Model file for the job. Use its own axes, mm. Face numbers are marked on the shaded views. Round coordinates to 2 decimals unless told otherwise and drop trailing zeros. Loops run counter-clockwise (first coordinate to the right, second up) from the corner with the lowest first, then second, coordinate; pieces in that order, holes last. Notation, with made-up numbers: M -26.75,36.5 L 6.25,36.5 A8 cw 6.25,41.5 Z; hole C -15.75,50 d10. An arc over 180 degrees is marked long. Use a Markdown table: item, result. Add a question column.
Q1. Mould opens along Z. For the marked faces 1 and 2 say: +Z half, -Z half, draft (parallel to the pull), parting line (faces both ways), or undercut.
Q2. Cut at B-B (z = 0). Give the cut face in (x, y), plus the area to 3 significant figures.
Q3. Probe line 1 (Z direction, x = -9, y = 4.25); line 2 (X direction, y = 4.7, z = 0); line 3 (Y direction, x = -38, z = -9). List the from-to ranges inside material, lowest first. Write a range as from..to.
Q4. Pin check, flat tips, straight feed: pin 1 (2.5 mm diameter, centred on y = 12, z = -6.5, fed in from +X); pin 2 (3.5 mm diameter, centred on x = -18.5, y = 4, fed in from -Z); pin 3 (5 mm diameter, centred on y = 3.5, z = 20, fed in from +X); pin 4 (1.5 mm diameter, centred on x = -40.5, z = -1, fed in from -Y). Stop position of each tip, or through.
Q5. Cut at A-A (x = 61.3). Give the cut face in (y, z), plus the area to 3 significant figures.
Q6. Cut at C-C (z = 61.3). Give the cut face in (x, y).
Q7. Cut at D-D (x = 0). Give the cut face in (y, z).
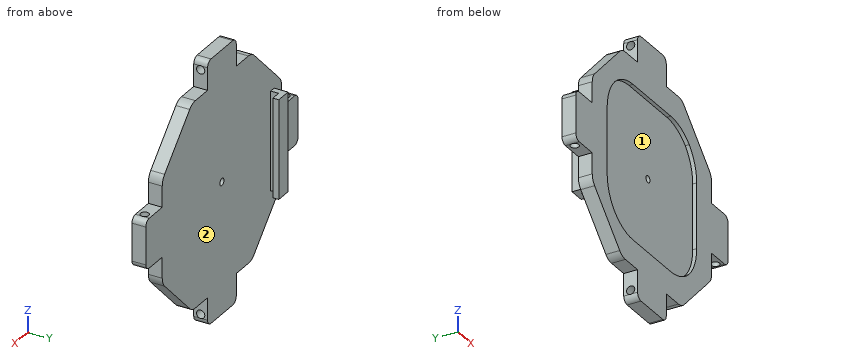
from build123d import *

# Parameters (mm, degrees)
SKETCH_1_W          = 14.3
SKETCH_1_H          = 25
SKETCH_1_W_2        = 25
SKETCH_1_H_2        = 14.3
EXTRUDE_1_DEPTH     = 7
FILLET_1_R          = 3
FILLET_2_R          = 7
FILLET_3_R          = 23
EXTRUDE_START       = -5
EXTRUDE_2_DEPTH     = 5
SKETCH_7_R          = 1.75
CUT_EXTRUDE_5_DEPTH = 95.023294986
SKETCH_9_W          = 3
SKETCH_9_H          = 50
EXTRUDE_3_DEPTH     = 7
SKETCH_10_W         = 50
SKETCH_10_H         = 3
EXTRUDE_4_DEPTH     = 5
SKETCH_11_R         = 2.1
CUT_EXTRUDE_6_DEPTH = 104.928485027
SKETCH_12_R         = 2.1
CUT_EXTRUDE_7_DEPTH = 104.928485103


with BuildPart() as part:
    # 스케치1 → 보스-돌출1 (new body)
    with BuildSketch(Plane(origin=(0, 0, 0), x_dir=(1, 0, 0), z_dir=(0, 1, 0))):
        Polygon((-26, 52), (-39, 39), (-26, 39), (26, 39), (39, 39), (26, 52), (12.5, 52), (-12.5, 52), align=None)
        Polygon((-26, 39), (-39, 39), (-39, 26), align=None)
        Polygon((-39, 26), (-39, 39), (-52, 26), (-52, 12.5), (-52, -12.5), (-52, -26), (-39, -39), (-39, -26), align=None)
        with Locations((-59.15, 0)):
            Rectangle(SKETCH_1_W, SKETCH_1_H)
        with Locations((0, 59.15)):
            Rectangle(SKETCH_1_W_2, SKETCH_1_H_2)
        Polygon((39, 39), (26, 39), (39, 26), align=None)
        Polygon((52, 26), (39, 39), (39, 26), (39, -26), (39, -39), (52, -26), (52, -12.5), (52, 12.5), align=None)
        with Locations((59.15, 0)):
            Rectangle(SKETCH_1_W, SKETCH_1_H)
        Polygon((39, -39), (39, -26), (26, -39), align=None)
        Polygon((-26, -39), (-39, -39), (-26, -52), (-12.5, -52), (12.5, -52), (26, -52), (39, -39), (26, -39), align=None)
        Polygon((-26, -39), (-39, -26), (-39, -39), align=None)
        with Locations((0, -59.15)):
            Rectangle(SKETCH_1_W_2, SKETCH_1_H_2)
    extrude(amount=EXTRUDE_1_DEPTH)

    # 필렛1
    fillet_1_edges = [part.edges().sort_by_distance(p)[0] for p in [
        (12.5, 3.5, 66.3),
        (-12.5, 3.5, 66.3),
        (-66.3, 3.5, 12.5),
        (-66.3, 3.5, -12.5),
        (-12.5, 3.5, -66.3),
        (12.5, 3.5, -66.3),
        (66.3, 3.5, -12.5),
        (66.3, 3.5, 12.5),
    ]]
    fillet(fillet_1_edges, radius=FILLET_1_R)

    # 필렛2
    fillet_2_edges = [part.edges().sort_by_distance(p)[0] for p in [
        (-26, 3.5, 52),
        (-52, 3.5, 26),
        (-52, 3.5, -26),
        (-26, 3.5, -52),
        (26, 3.5, -52),
        (52, 3.5, -26),
        (52, 3.5, 26),
        (26, 3.5, 52),
    ]]
    fillet(fillet_2_edges, radius=FILLET_2_R)

    # 필렛3
    # the kernel refuses this fillet: 23 mm, written as the material it adds along each edge
    with BuildSketch(Plane(origin=(-39, 0, 26), x_dir=(0, 0, -1), z_dir=(0, 1, 0))) as fillet_3_piece_1:
        with BuildLine():
            CenterArc((FILLET_3_R * 0.414213562373, -FILLET_3_R), FILLET_3_R, 90, 45)
            Line((-FILLET_3_R * 0.292893218813, -FILLET_3_R * 0.292893218813), (0, 0))
            Line((0, 0), (FILLET_3_R * 0.414213562373, 0))
        make_face()
    extrude(amount=7)
    with BuildSketch(Plane(origin=(-26, 0, 39), x_dir=(1, 0, 0), z_dir=(0, 1, 0)), Plane(origin=(26, 0, 39), x_dir=(0.7071067811865479, 0, -0.7071067811865471), z_dir=(0, 1, 0)), Plane(origin=(39, 0, 26), x_dir=(0, 0, -1), z_dir=(0, 1, 0)), Plane(origin=(39, 0, -26), x_dir=(-0.7071067811865476, 0, -0.7071067811865476), z_dir=(0, 1, 0)), Plane(origin=(26, 0, -39), x_dir=(-1, 0, 0), z_dir=(0, 1, 0)), Plane(origin=(-26, 0, -39), x_dir=(-0.7071067811865471, 0, 0.7071067811865479), z_dir=(0, 1, 0)), Plane(origin=(-39, 0, -26), x_dir=(0, 0, 1), z_dir=(0, 1, 0))) as fillet_3_piece_2:
        with BuildLine():
            CenterArc((FILLET_3_R * 0.414213562373, FILLET_3_R), FILLET_3_R, 225, 45)
            Line((-FILLET_3_R * 0.292893218813, FILLET_3_R * 0.292893218813), (0, 0))
            Line((0, 0), (FILLET_3_R * 0.414213562373, 0))
        make_face()
    extrude(amount=7)

    # 스케치6 → 보스-돌출2 (add)
    with BuildSketch(Plane(origin=(0, 7, 0), x_dir=(1, 0, 0), z_dir=(0, 1, 0)).offset(EXTRUDE_START)):
        with BuildLine():
            Line((16.473088065, 39), (-16.473088065, 39))
            ThreePointArc((-16.473088065, 39), (-25.120040329, 37.312677367), (-32.4982797, 32.4982797))
            ThreePointArc((-32.4982797, 32.4982797), (-37.312677367, 25.120040329), (-39, 16.473088065))
            Line((-39, 16.473088065), (-39, -16.473088065))
            ThreePointArc((-39, -16.473088065), (-37.312677367, -25.120040329), (-32.4982797, -32.4982797))
            ThreePointArc((-32.4982797, -32.4982797), (-25.120040329, -37.312677367), (-16.473088065, -39))
            Line((-16.473088065, -39), (16.473088065, -39))
            ThreePointArc((16.473088065, -39), (25.120040329, -37.312677367), (32.4982797, -32.4982797))
            ThreePointArc((32.4982797, -32.4982797), (37.312677367, -25.120040329), (39, -16.473088065))
            Line((39, -16.473088065), (39, 16.473088065))
            ThreePointArc((39, 16.473088065), (37.312677367, 25.120040329), (32.4982797, 32.4982797))
            ThreePointArc((32.4982797, 32.4982797), (25.120040329, 37.312677367), (16.473088065, 39))
        make_face()
    extrude(amount=EXTRUDE_2_DEPTH)

    # 스케치7 → 컷-돌출5 (cut, through all)
    with BuildSketch(Plane(origin=(0, 7, 0), x_dir=(1, 0, 0), z_dir=(0, 1, 0))):
        with Locations(Location((0, 0, 0), (0, 0, 270))):
            Circle(SKETCH_7_R)
    extrude(amount=-CUT_EXTRUDE_5_DEPTH, mode=Mode.SUBTRACT)

    # 스케치9 → 보스-돌출3 (add)
    with BuildSketch(Plane(origin=(0, 7, 0), x_dir=(1, 0, 0), z_dir=(0, 1, 0))):
        with Locations((-44, 0)):
            Rectangle(SKETCH_9_W, SKETCH_9_H)
    extrude(amount=EXTRUDE_3_DEPTH)

    # 스케치10 → 보스-돌출4 (add)
    with BuildSketch(Plane(origin=(-42.5, 0, 0), x_dir=(0, 0, -1), z_dir=(1, 0, 0))):
        with Locations((0, 12.5)):
            Rectangle(SKETCH_10_W, SKETCH_10_H)
    extrude(amount=EXTRUDE_4_DEPTH)

    # 스케치11 → 컷-돌출6 (cut, through all)
    with BuildSketch(Plane.XY.offset(12.5)):
        with Locations(Location((-61.3, 3.5, 0), (0, 0, 197.752790162))):
            Circle(SKETCH_11_R)
        with Locations(Location((61.3, 3.5, 0), (0, 0, 17.752790162))):
            Circle(SKETCH_11_R)
    extrude(amount=-CUT_EXTRUDE_6_DEPTH, mode=Mode.SUBTRACT)

    # 스케치12 → 컷-돌출7 (cut, through all)
    with BuildSketch(Plane.ZY.offset(12.5)):
        with Locations(Location((-61.3, 3.5, 0), (0, 0, 162.247209838))):
            Circle(SKETCH_12_R)
        with Locations(Location((61.3, 3.5, 0), (0, 0, 17.752790162))):
            Circle(SKETCH_12_R)
    extrude(amount=-CUT_EXTRUDE_7_DEPTH, mode=Mode.SUBTRACT)


solid = part.part
Checked values:
| question | item | result |
|---|---|---|
| 1 | face 1 | undercut |
| 1 | face 2 | draft |
| 2 | outline | M -66.3,0 L -39,0 L -39,2 L -1.75,2 L -1.75,7 L -42.5,7 L -42.5,11 L -37.5,11 L -37.5,14 L -45.5,14 L -45.5,7 L -66.3,7 Z; M 1.75,2 L 39,2 L 39,0 L 66.3,0 L 66.3,7 L 1.75,7 Z; hole C -61.3,3.5 d4.2; hole C 61.3,3.5 d4.2 |
| 2 | area | 763 mm^2 |
| 3 | line 1 | z = -66.3..-63.26, -59.34..59.34, 63.26..66.3 |
| 3 | line 2 | x = -66.3..-63.02, -59.58..-1.75, 1.75..59.58, 63.02..66.3 |
| 3 | line 3 | y = 2..7, 11..14 |
| 4 | pin 1 | stops at x = -37.5 |
| 4 | pin 2 | stops at z = -52 |
| 4 | pin 3 | stops at x = 52 |
| 4 | pin 4 | stops at y = 0 |
| 5 | outline | M 0,-12.5 L 1.4,-12.5 L 1.4,12.5 L 0,12.5 Z; M 5.6,-12.5 L 7,-12.5 L 7,12.5 L 5.6,12.5 Z |
| 5 | area | 70.0 mm^2 |
| 6 | outline | M -12.5,0 L 12.5,0 L 12.5,1.4 L -12.5,1.4 Z; M -12.5,5.6 L 12.5,5.6 L 12.5,7 L -12.5,7 Z |
| 7 | outline | M 0,-66.3 L 7,-66.3 L 7,-1.75 L 2,-1.75 L 2,-39 L 0,-39 Z; M 0,39 L 2,39 L 2,1.75 L 7,1.75 L 7,66.3 L 0,66.3 Z; hole C 3.5,-61.3 d4.2; hole C 3.5,61.3 d4.2 |
